from build123d import *

# Parameters (mm, degrees)
F1_DEPTH = 7
F2_W     = 5
F2_H     = 7
F2_W_2   = 7
F2_H_2   = 5
F3_DEPTH = 7.001
F5_DEPTH = 7.001


with BuildPart() as f1:
    # F0 (on Top) → F1 (new body)
    with BuildSketch(Plane.XY):
        with BuildLine():
            Line((-85, -75), (85, -75))
            Line((85, -75), (85, -40))
            ThreePointArc((85, -40), (54.689259, -64.429409), (37.256318, -29.620939))
            Line((37.256318, -29.620939), (85, 75))
            Line((85, 75), (60, 75))
            Line((60, 75), (45.469314, 43.158845))
            Line((45.469314, 43.158845), (-45.469314, 43.158845))
            Line((-45.469314, 43.158845), (-60, 75))
            Line((-60, 75), (-85, 75))
            Line((-85, 75), (-37.256318, -29.620939))
            ThreePointArc((-37.256318, -29.620939), (-35.570591, -34.689259), (-35, -40))
            ThreePointArc((-35, -40), (-60, -65), (-85, -40))
            Line((-85, -40), (-85, -75))
        make_face()
    extrude(amount=F1_DEPTH)

    # F2 (on face) → F3 (cut, through all)
    with BuildSketch(Plane.XY.offset(7)):
        with Locations((-30, -65)):
            Rectangle(F2_W, F2_H)
        with Locations((30, -65)):
            Rectangle(F2_W, F2_H)
        with Locations((-30, -40)):
            Rectangle(F2_W, F2_H)
        with Locations((30, -40)):
            Rectangle(F2_W, F2_H)
        with Locations((-30, 0)):
            Rectangle(F2_W_2, F2_H_2)
        with Locations((30, 0)):
            Rectangle(F2_W_2, F2_H_2)
    extrude(amount=-F3_DEPTH, mode=Mode.SUBTRACT)

    # F4 (on face) → F5 (cut, through all)
    with BuildSketch(Plane.XY.offset(7)):
        Polygon((71.213039, 62.853791), (75.761776, 60.777978), (78.667913, 67.146209), (74.119177, 69.222022), align=None)
        Polygon((52.959071, 22.853791), (57.507808, 20.777978), (60.413945, 27.146209), (55.865208, 29.222022), align=None)
        Polygon((-57.507808, 20.777978), (-52.959071, 22.853791), (-55.865208, 29.222022), (-60.413945, 27.146209), align=None)
        Polygon((-75.761776, 60.777978), (-71.213039, 62.853791), (-74.119177, 69.222022), (-78.667913, 67.146209), align=None)
    extrude(amount=-F5_DEPTH, mode=Mode.SUBTRACT)


solid = f1.part
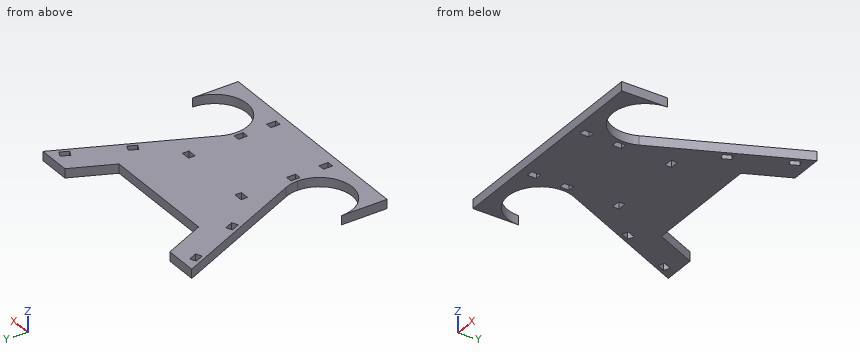
Could you check a few things on this model? Use its own coordinates, in mm. Round coordinates to 2 decimals unless told otherwise and drop trailing zeros. Write each loop counter-clockwise with the first axis right and the second up, starting at its lowest first coordinate (ties: lowest second). Pieces come first, ordered by that corner, then holes. Notation, with made-up numbers: (87, 8.5) - (104, 8.5) arc R12 ccw to (104, 13.5) - close; hole circle Ø4 at (-23, -13). An arc over 180 degrees is marked (long way). Put each result on its own line as item: value. Start each with the question number.
(1) I want a section at B-B, the plane y = 48. Please give me the cut outline in (x, z).
(2) I want a section at C-C, the plane z = 1.25. Give the number of separate pieces and of enclosed holes in the cut face, plus the area to 3 significant figures.
(3) I want a section at A-A, the plane x = -64. Please give me the cut outline in (y, z).
(4) I need wall thicknesses on probe 1 along Y at (x, z) = (-28, 2); probe 2 along Y at (x, z) = (60, 2.5); probe 3 along Y at (x, z) = (73, 6). Which ranges of each line are inside material? Lowest first, please.
(5) I want a section at D-D, the plane x = 5.5. Please give me the cut outline in (y, z).
(6) Will these pins go through, and if not, where does the flat tip stop? pin 1 (4 mm diameter, centred on x = -30, z = 3, fed in from +Y); pin 2 (4 mm diameter, centred on y = 1, z = 4.5, fed in from +X).
Here are the results:
1. outline: (-72.68, 0) - (-47.68, 0) - (-47.68, 7) - (-72.68, 7) - close; (47.68, 0) - (72.68, 0) - (72.68, 7) - (47.68, 7) - close
2. separate pieces: 1
2. enclosed holes: 10
2. area: 13,800 mm^2
3. outline: (-75, 0) - (-64.68, 0) - (-64.68, 7) - (-75, 7) - close; (28.98, 0) - (75, 0) - (75, 7) - (28.98, 7) - close
4. probe 1: y = -75 to -68.5, -61.5 to -43.5, -36.5 to -2.5, 2.5 to 43.16
4. probe 2: y = -75 to -65, 20.22 to 26.24, 27.34 to 75
4. probe 3: y = -75 to -61.35, 48.7 to 62.04, 66.77 to 75
5. outline: (-75, 0) - (43.16, 0) - (43.16, 7) - (-75, 7) - close
6. pin 1: stops at y = 43.16
6. pin 2: stops at x = 52.14
